Check sheet for the modelled part. Datum: model origin and axes. Units: mm. A direction names the side the tool comes from. Coordinates: 2 decimals unless noted, no trailing zeros. Write each loop counter-clockwise with the first axis right and the second up, starting at its lowest first coordinate (ties: lowest second). Pieces come first, ordered by that corner, then holes. Notation, with made-up numbers: (85, 23.5) - (108, 23.5) arc R17 ccw to (108, 54.5) - close; hole circle Ø2 at (-20.75, -12). An arc over 180 degrees is marked (long way). Answer as CSV lines item,"result". Start each with the question number.
from build123d import *

# Parameters (mm, degrees)
SKETCH1_W                 = 160
SKETCH1_H                 = 50.8
BOSS_EXTRUDE1_DEPTH       = 10
SKETCH2_R                 = 6.35
BOSS_EXTRUDE2_DEPTH       = 160
SKETCH3_W                 = 27
SKETCH3_H                 = 40
SKETCH3_W_2               = 18
SKETCH3_W_3               = 25
CUT_EXTRUDE2_DEPTH        = 176.158899289
F_4_0_25_DIAMETER_HOLE1_D = 6.35


with BuildPart() as part:
    # Sketch1 → Boss-Extrude1 (new body)
    with BuildSketch(Plane(origin=(0, 0, 0), x_dir=(1, 0, 0), z_dir=(0, 1, 0))):
        with Locations((80, 25.4)):
            Rectangle(SKETCH1_W, SKETCH1_H)
    extrude(amount=BOSS_EXTRUDE1_DEPTH)

    # Sketch2 → Boss-Extrude2 (add, through all)
    with BuildSketch(Plane.ZY):
        with BuildLine():
            Line((-50.8, 10), (-39.444175854, 40.268882668))
            ThreePointArc((-39.444175854, 40.268882668), (-25.4, 50), (-11.355824146, 40.268882668))
            Line((-11.355824146, 40.268882668), (0, 10))
            Line((0, 10), (-50.8, 10))
        make_face()
        with Locations((-25.4, 35)):
            Circle(SKETCH2_R, mode=Mode.SUBTRACT)
    extrude(amount=-BOSS_EXTRUDE2_DEPTH)

    # Sketch3 → Cut-Extrude2 (cut, through all)
    with BuildSketch(Plane(origin=(0, 0, -50.8), x_dir=(-1, 0, 0), z_dir=(0, 0, -1))):
        with Locations((-13.5, 30)):
            Rectangle(SKETCH3_W, SKETCH3_H)
        with Locations((-50, 30)):
            Rectangle(SKETCH3_W_2, SKETCH3_H)
        with Locations((-82, 30)):
            Rectangle(SKETCH3_W_2, SKETCH3_H)
        with Locations((-114, 30)):
            Rectangle(SKETCH3_W_2, SKETCH3_H)
        with Locations((-147.5, 30)):
            Rectangle(SKETCH3_W_3, SKETCH3_H)
    extrude(amount=-CUT_EXTRUDE2_DEPTH, mode=Mode.SUBTRACT)

    # #4 (0.25) Diameter Hole1 (through all)
    with Locations(Plane(origin=(0, 10, 0), x_dir=(1, 0, 0), z_dir=(0, 1, 0))):
        with Locations((82.5, 38.1), (82.5, 12.7), (147, 12.7), (147, 38.1), (13, 38.1), (13, 12.7)):
            Hole(F_4_0_25_DIAMETER_HOLE1_D / 2)


solid = part.part
(1) Go/stop test with flat-tipped pins: P1, Ø1.5, axis at x = 132.5, y = 32.5, coming from the +Z side; P2, Ø8.5, axis at x = 147, z = -38.1, coming from the +Y side; P3, Ø8, axis at x = 119.5, y = 17, coming from the -Z side. Record where each tip stops, or that it passes through.
(2) Cross-section at D-D on y = 14.5. Record the boundary of the cut face in (x, z).
(3) Cross-section at C-C on x = 127.5. Record the boundary of the cut face in (y, z).
(4) Material ranges on probe 1 along Z at (x, y) = (13, 3) (3 decimals); probe 2 along X at (y, z) = (3, -12.7) (3 decimals); probe 3 along X at (y, z) = (19, -26), recorded low to high. Write a range as from..to.
(5) Tool access check on faces 4 (the face through (91, 25, -26)), 5 (the face through (79.47, 4.93, -39.05)), 6 (the face through (27, 25, -26)). Record the directions out of +Z, -Z, +X, -X, +Y, -Y that give a thin tool (end or side, any length) a straight path to the whole face; none if there is none.
(6) Cross-section at B-B on y = 7. Record the boundary of the cut face in (x, z) (3 decimals).
(7) Cross-section at A-A on x = 82.5. Record the boundary of the cut face in (y, z) (3 decimals), plus the area to 3 significant figures.
(8) Release check for a two-part mould opening along Z. For faces 1 (the face through (97.9, 41.3, -26.2)), 2 (the face through (97.902, 24.923, -45.202)), 3 (the face through (14, 10, -26)) record: pulls with the +Z half, pulls with the -Z half, needs draft (parallel to the pull), parting line crosses it, or undercut.
Checked values:
1,P1,"z = -8.16"
1,P2,"y = 10"
1,P3,"z = -48.9"
2,outline,"(27, -49.11) - (41, -49.11) - (41, -1.69) - (27, -1.69) - close; (59, -49.11) - (73, -49.11) - (73, -1.69) - (59, -1.69) - close; (91, -49.11) - (105, -49.11) - (105, -1.69) - (91, -1.69) - close; (123, -49.11) - (135, -49.11) - (135, -1.69) - (123, -1.69) - close"
3,outline,"(0, -50.8) - (10, -50.8) - (40.27, -39.44) arc R15 ccw to (40.27, -11.36) - (10, 0) - (0, 0) - close; hole circle Ø12.7 at (35, -25.4)"
4,probe 1,"-50.8..-41.275, -34.925..-15.875, -9.525..0"
4,probe 2,"0..9.825, 16.175..79.325, 85.675..143.825, 150.175..160"
4,probe 3,"27..41, 59..73, 91..105, 123..135"
5,face 4,"+Z, -Z, +Y"
5,face 5,"+Y, -Y"
5,face 6,"+Z, -Z, -X, +Y"
6,outline,"(0, -50.8) - (160, -50.8) - (160, 0) - (0, 0) - close; hole circle Ø6.35 at (13, -38.1); hole circle Ø6.35 at (13, -12.7); hole circle Ø6.35 at (82.5, -38.1); hole circle Ø6.35 at (82.5, -12.7); hole circle Ø6.35 at (147, -38.1); hole circle Ø6.35 at (147, -12.7)"
7,outline,"(0, -50.8) - (10, -50.8) - (10, -41.275) - (0, -41.275) - close; (0, -34.925) - (10, -34.925) - (10, -15.875) - (0, -15.875) - close; (0, -9.525) - (10, -9.525) - (10, 0) - (0, 0) - close"
7,area,"381 mm^2"
8,face 1,"undercut"
8,face 2,"pulls with the -Z half"
8,face 3,"needs draft"
